Study the drawing (mm; zero at the part's minimum x, y, z) and answer. A direction names the side the tool comes from. Round coordinates to 2 decimals unless told otherwise and drop trailing zeros. Write each loop counter-clockwise with the first axis right and the second up, starting at its lowest first coordinate (ties: lowest second). Pieces come first, ordered by that corner, then holes. Notation, with made-up numbers: (17.5, 74) -> (24.5, 74) arc R32 cw to (24.5, 109) -> close; hole circle Ø1 at (67, 23). An arc over 180 degrees is marked (long way). One line per question, with ' | ' between items. Start each with the question number.
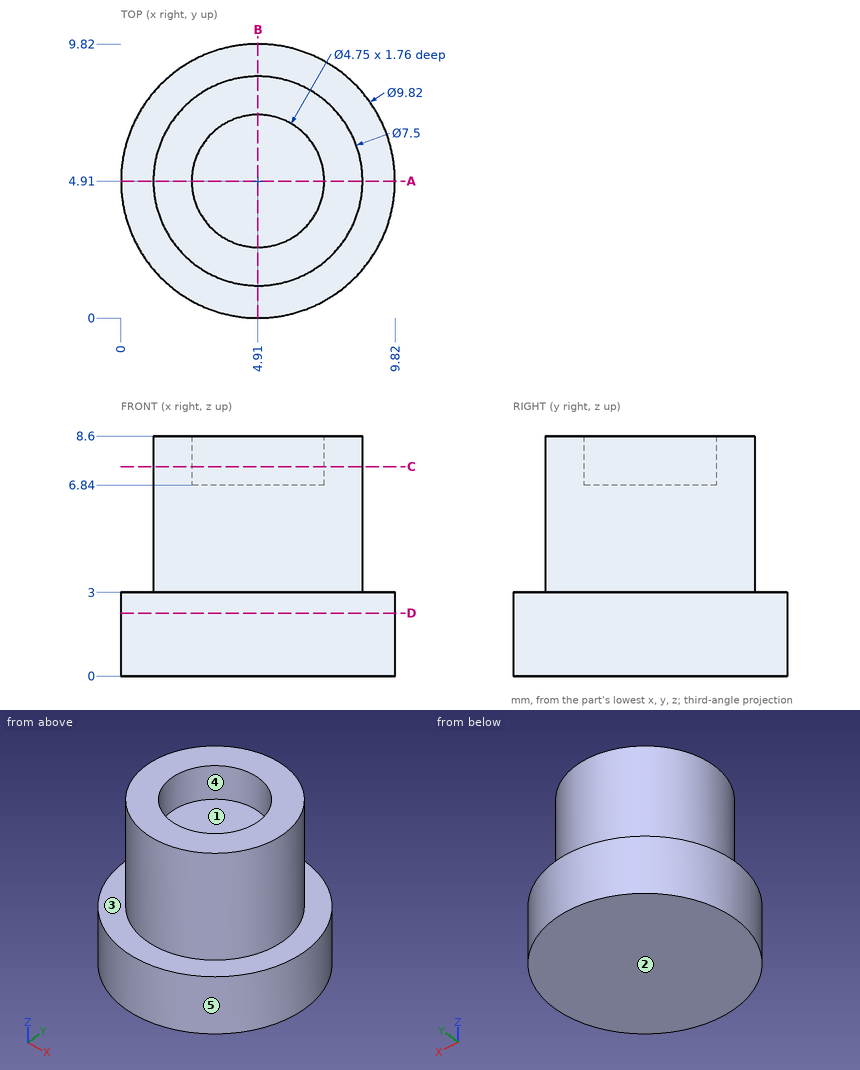
(1) A cutting plane is placed at C-C, the plane z = 7.5. Determine the outline of the cut face in (x, y) (3 decimals), then the cut area to 3 significant figures.
(2) Consider L1, parallel to Y at x = 4.91, z = 7.8 (3 decimals); L2, parallel to Z at x = 3.25, y = 6; L3, parallel to Z at x = 8.5, y = 6.5. Determine where each line is inside the solid, lowest interval first.
(3) The mould has two halves that part along X. Classify the marked faces 3, 4 and 5: +X half, -X half, draft (parallel to the pull), parting line (faces both ways), or undercut.
(4) A cutting plane is placed at D-D, the plane z = 2.25. Determine the outline of the cut face in (x, y), then the cut area to 3 significant figures.
(5) Given pin 1 Ø1.4 at (x, y) = (5, 5.5) entering from +Z; pin 2 Ø1 at (x, z) = (1.5, 3) entering from -Y, each flat-ended and moving along its own axis, determine where each tip first touches the part or whether it passes through.
(6) For the marked faces 1 and 2, determine the directions among +Z, -Z, +X, -X, +Y, -Y from which every point of the face is accessible in a straight line to the end or side of a thin tool.
(7) A cutting plane is placed at A-A, the plane y = 4.91. Determine the outline of the cut face in (x, z) (3 decimals), then the cut area to 3 significant figures.
Returned:
1) outline: circle Ø7.5 at (4.91, 4.91); hole circle Ø4.75 at (4.91, 4.91) | area: 26.5 mm2
2) L1: 1.16 to 2.535, 7.285 to 8.66 | L2: 0 to 6.84 | L3: 0 to 3
3) face 3: draft | face 4: undercut | face 5: parting line
4) outline: circle Ø9.82 at (4.91, 4.91) | area: 75.7 mm2
5) pin 1: z = 6.84 | pin 2: y = 0.96
6) face 1: +Z | face 2: -Z, +X, -X, +Y, -Y
7) outline: (0, 0) -> (9.82, 0) -> (9.82, 3) -> (8.66, 3) -> (8.66, 8.6) -> (7.285, 8.6) -> (7.285, 6.84) -> (2.535, 6.84) -> (2.535, 8.6) -> (1.16, 8.6) -> (1.16, 3) -> (0, 3) -> close | area: 63.1 mm2
